Build history of the part. All positions in model axes, mm. A direction names the side the tool comes from. Round coordinates to 2 decimals unless told otherwise and drop trailing zeros. Write each loop counter-clockwise with the first axis right and the second up, starting at its lowest first coordinate (ties: lowest second). Pieces come first, ordered by that corner, then holes. Notation, with made-up numbers: (2, -3) - (23, -3) arc R29 ccw to (23, 34) - close; hole circle Ø7 at (80, 72.5). An arc over 180 degrees is marked (long way). One line per question, with ' | ' between items.
Autodesk Inventor part; units mm, degrees
ref_plane "YZ Plane" through (0, 0, 0) normal (1, 0, 0) x (0, 1, 0)
ref_plane "XZ Plane" through (0, 0, 0) normal (0, 1, 0) x (-1, 0, 0)
ref_plane "XY Plane" through (0, 0, 0) normal (0, 0, 1) x (1, 0, 0)
sketch "Эскиз1" plane through (0, 0, 0) normal (0, 1, 0) x (-1, 0, 0)
  circle A0 centre (0, 0) radius 2.45
  circle A1 centre (0, 0) radius 3.75
  dimension "d0" = 4.9
  dimension "d1" = 7.5
extrude "Выдавливание1" add sketch "Эскиз1" along normal blind 6
sketch "Эскиз2" plane through (0, 0, 0) normal (1, 0, 0) x (0, 1, 0)
  circle A0 centre (3, 0) radius 1.25
  line L0 (0, -3.75) -> (0, 3.75)
  circle A1 centre (3, 0) radius 3
  circle A2 centre (3, 7.071) radius 1.25
  arc A3 (6, 7.071) -> (0, 7.071) centre (3, 7.071) ccw
  line L1 (3, 0) -> (3, 7.071) construction
  line L2 (6, 0) -> (6, 7.071)
  line L3 (0, 7.071) -> (0, 0)
  point P0 (0, 0)
  dimension "d7" = 6
  dimension "d4" = 2.5
  dimension "d12" = 2.5
  dimension "d13" = 6
  dimension "d14" = 7.071
extrude "Выдавливание3" add sketch "Эскиз2" along normal mid plane 7.5 contours A1
extrude "Выдавливание5" add sketch "Эскиз2" along normal blind 1.85 and the other way blind 3.75 contours L0 L3 A3 L2 A1
extrude "Выдавливание2" add sketch "Эскиз2" along normal mid plane 11 contours A0
extrude "Выдавливание4" cut sketch "Эскиз1" along normal blind 6 contours A0
extrude "Выдавливание7" add sketch "Эскиз2" along normal blind 3.6 and the other way blind 5.5 contours A2
sketch "Эскиз3" plane through (1.85, 0, 0) normal (1, 0, 0) x (0, 0, -1)
  circle A0 centre (-7.071, 3) radius 1.25
  line L0 (-4.4382, 1.5618) -> (0, 6)
  line L1 (-3.2619, 6) -> (-7.071, 6)
  line L2 (0, 6) -> (-3.2619, 6)
  arc A1 (-7.071, 6) -> (-7.071, 0) centre (-7.071, 3) ccw
  arc A2 (-7.071, 0) -> (-7.071, 6) centre (-7.071, 3) ccw
  line L3 (3.75, 6) -> (0, 6)
  point P0 (0, 0)
  dimension "d26" = 45
extrude "Выдавливание8" cut sketch "Эскиз3" along normal blind 3.75 contours A2 L1 L2 L0
properties part number "Кулак левый"
Q1. Saw through at A-A, the plane x = 0. List the corners of the cut face in (y, z), then the cut area to 3 significant figures.
Found:
outline: (0, -3.75) - (6, -3.75) - (6, -2.45) - (0, -2.45) - close; (0, 2.45) - (6, 2.45) - (6, 7.07) arc R3 ccw to (0, 7.07) - close | area: 49.7 mm^2
Q2. Drop flat-ended pins along their axis: pin 1 (1 mm diameter, centred on x = 2.5, y = 1, fed in from -Z); pin 2 (0.8 mm diameter, centred on y = 2.5, z = 6.5, fed in from +X); pin 3 (1.5 mm diameter, centred on y = 5, z = 8, fed in from -X). Give the stop position or say it passes through.
Found:
pin 1: z = -3.17 | pin 2: x = 3.6 | pin 3: x = -3.75
Q3. Pull direction X, two halves, no side cores. Call faces 1 (the flat face through (-5.5, 3, 0)), 2 (the flat face through (3.6, 3, 7)), 3 (the cylindrical face through (-2.337, 2.958, -0.736)): +X half, -X half, draft (parallel to the pull), parting line (faces both ways), or undercut.
Found:
face 1: -X half | face 2: +X half | face 3: undercut
Q4. Which spindle directions (+Z, -Z, +X, -X, +Y, -Y) get a long thin tool onto all of the face, cutting with end or side? Do faces 4 (the cylindrical face through (-3, 3, -3)), 5 (the cylindrical face through (-4.613, 3.577, 5.962)), 6 (the cylindrical face through (-0.08, 2.96, -3.75)). Say none if no direction does.
Found:
face 4: -Z, -X | face 5: -X | face 6: -Z
Q5. Saw through at B-B, the plane z = -1.5. List the corners of the cut face in (x, y), then the cut area to 3 significant figures.
Found:
outline: (-3.75, 0.4) - (-3.44, 0.4) - (-3.44, 0) - (-1.94, 0) - (-1.94, 6) - (-3.44, 6) - (-3.44, 5.6) - (-3.75, 5.6) - close; (1.94, 0) - (3.44, 0) - (3.44, 0.4) - (3.75, 0.4) - (3.75, 5.6) - (3.44, 5.6) - (3.44, 6) - (1.94, 6) - close | area: 21.3 mm^2
Q6. Saw through at C-C, the plane y = 1. List the corners of the cut face in (x, z), then the cut area to 3 significant figures.
Found:
outline: (-3.75, -2.24) - (-3.01, -2.24) arc R3.75 ccw to (3.01, -2.24) - (3.75, -2.24) - (3.75, 2.24) - (3.01, 2.24) arc R3.75 ccw to (1.85, 3.26) - (1.85, 9.31) - (-3.75, 9.31) - close; hole circle Ø4.9 at (0, 0) | area: 61.3 mm^2
Q7. Saw through at D-D, the plane z = 4.25. List the corners of the cut face in (x, y), then the cut area to 3 significant figures.
Found:
outline: (-3.75, 0) - (1.85, 0) - (1.85, 6) - (-3.75, 6) - close | area: 33.6 mm^2
Q8. Drill centre lines: L1, parallel to X at y = 4.1, z = 0; L2, parallel to Z at x = 0, y = 2.85; L3, parallel to X at y = 2, z = 6.5. Where is each one in solid material? Low to high. Write a range as from..to.
Found:
L1: -5.5..-2.45, 2.45..5.5 | L2: -3.75..-2.45, 2.45..10.07 | L3: -5.5..3.6
